Read the model definition and answer for the solid it produces. Units are mm, in the model's axes. A direction names the side the tool comes from. Coordinates: 2 decimals unless noted, no trailing zeros. Write each loop counter-clockwise with the first axis right and the second up, starting at its lowest first coordinate (ties: lowest second). Pieces come first, ordered by that corner, then holes.
Item 1: Section C-C (z = 7) is taken. Give the vertices of the cut face in (x, y), then the cut area to 3 significant figures.
Item 2: Section A-A (y = -35) is taken. Give the vertices of the cut face in (x, z), then the cut area to 3 significant figures.
Item 3: Straight lines are drawn through the part: probe 1 along X at (y, z) = (-47.25, 35); probe 2 along X at (y, z) = (-39.65, 35); probe 3 along X at (y, z) = (-4.5, 49.5). For each, find the intervals that lie inside material, in ascending order.
Item 4: Each of these flat-tipped pins is pushed along its axis until it touches: P1, Ø14.5, axis at x = 87, z = 27, coming from the +Y side; P2, Ø10, axis at y = -14, z = 15, coming from the -X side; P3, Ø3, axis at y = -5, z = 38.5, coming from the -X side. Where does it stop, or does it pass through?
Item 5: A tool of negligible diameter and unlimited length cuts with its end or side. For faces 1 (the face through (75, -12, 24)), 2 (the face through (95, -41, 37)), 3 (the face through (59.71, -30.906, 5.354)), 4 (the face through (28, -42, 35)), from which of +Z, -Z, +X, -X, +Y, -Y can it reach the whole face along a straight path? Write none if from no direction.
Item 6: Determine the mould class of faces 5 (the face through (22, -25, 0)), 6 (the face through (21.445, -24.65, 14.021)), 7 (the face through (54.284, -46.056, 29.06)), 8 (the face through (60, -26, 55)) for opening direction Z: released by +Z, released by -Z, zero draft, split by the parting line, or undercut.
from build123d import *

# Parameters (mm, degrees)
F0_W      = 100
F0_H      = 63
F1_DEPTH  = 50
F2_W      = 40
F2_H      = 15
F3_DEPTH  = 50
F5_DEPTH  = 9
F6_R      = 10
F7_W      = 50
F7_H      = 12
F8_DEPTH  = 48.001
F10_DEPTH = 50
F11_R     = 25
F12_DEPTH = 8
F13_R     = 24.9809
F13_R_2   = 10
F14_DEPTH = 5
F15_R     = 5
F16_DEPTH = 8
F18_DEPTH = 70.001


with BuildPart() as f1:
    # F0 (on Front) → F1 (new body)
    with BuildSketch(Plane.XZ):
        with Locations((50, 31.5)):
            Rectangle(F0_W, F0_H)
    extrude(amount=F1_DEPTH)

    # F2 (on face) → F3 (cut, through all)
    with BuildSketch(Plane.XZ.offset(50)):
        with Locations((80, 55.5)):
            Rectangle(F2_W, F2_H)
        Polygon((80, 12.7389581993), (45, 0), (92.7389581993, 0), align=None)
    extrude(amount=-F3_DEPTH, mode=Mode.SUBTRACT)

    # F4 (on face) → F5 (cut)
    with BuildSketch(Plane.XZ.offset(50)):
        with BuildLine():
            Line((100, 25), (100, 48))
            Line((100, 48), (90, 48))
            Line((90, 48), (90, 35))
            ThreePointArc((90, 35), (92.9289321881, 27.9289321881), (100, 25))
        make_face()
    extrude(amount=-F5_DEPTH, mode=Mode.SUBTRACT)

    # F6
    f6_edges = [f1.edges().sort_by_distance(p)[0] for p in [
        (80, -25, 12.738958),
    ]]
    fillet(f6_edges, radius=F6_R)

    # F7 (on face) → F8 (cut, through all)
    with BuildSketch(Plane.XY.offset(48)):
        with Locations((75, -6)):
            Rectangle(F7_W, F7_H)
    extrude(amount=-F8_DEPTH, mode=Mode.SUBTRACT)

    # F9 (on face) → F10 (cut, through all)
    with BuildSketch(Plane(origin=(0, 0, 0), x_dir=(-1, 0, 0), z_dir=(0, 1, 0))):
        with BuildLine():
            Line((-30, 63), (-30, 35))
            ThreePointArc((-30, 35), (-21.2132034356, 13.7867965644), (0, 5))
            Line((0, 5), (0, 63))
            Line((0, 63), (-30, 63))
        make_face()
    extrude(amount=-F10_DEPTH, mode=Mode.SUBTRACT)

    # F11 (on face) → F12 (cut)
    with BuildSketch(Plane.XZ.offset(50)):
        with Locations((30, 35)):
            Circle(F11_R)
    extrude(amount=-F12_DEPTH, mode=Mode.SUBTRACT)

    # F13 (on face) → F14 (cut)
    with BuildSketch(Plane.XZ.offset(42)):
        with Locations((30, 35)):
            Circle(F13_R)
        with Locations((30, 35)):
            Circle(F13_R_2, mode=Mode.SUBTRACT)
    extrude(amount=-F14_DEPTH, mode=Mode.SUBTRACT)

    # F15 (on face) → F16 (join, through all)
    with BuildSketch(Plane.XZ.offset(42)):
        with Locations((30, 35)):
            Circle(F15_R)
    extrude(amount=F16_DEPTH)

    # F17 (on face) → F18 (cut, through all)
    with BuildSketch(Plane(origin=(30, 0, 0), x_dir=(0, -1, 0), z_dir=(-1, 0, 0))):
        Polygon((6.5514642168, 63), (0, 63), (0, 45), align=None)
    extrude(amount=-F18_DEPTH, mode=Mode.SUBTRACT)


solid = f1.part
Established:
1. outline: (10.77, -50) - (64.23, -50) - (64.23, -12) - (50, -12) - (50, 0) - (10.77, 0) - close; (85.74, -50) - (100, -50) - (100, -12) - (85.74, -12) - close
1. area: 3,040 mm2
2. outline: (0, 0) - (45, 0) - (74.01, 10.56) arc R10 cw to (84.5, 8.23) - (92.74, 0) - (100, 0) - (100, 48) - (60, 48) - (60, 63) - (30, 63) - (30, 35) arc R30 cw to (0, 5) - close
2. area: 3,860 mm2
3. probe 1: x = 25 to 35, 55 to 90
3. probe 2: x = 30 to 40, 54.98 to 100
3. probe 3: x = 30 to 60
4. P1: stops at y = -12
4. P2: stops at x = 16.58
4. P3: stops at x = 30
5. face 1: -Z, +X, +Y
5. face 2: +Z, +X, -Y
5. face 3: -Z, +Y, -Y
5. face 4: +Z, -X, +Y
6. face 5: released by -Z
6. face 6: released by +Z
6. face 7: undercut
6. face 8: zero draft
